from build123d import *

# Parameters (mm, degrees)
SKETCH1_R           = 30
SKETCH1_R_2         = 10
BOSS_EXTRUDE1_DEPTH = 6
CUT_EXTRUDE1_START  = -6
CUT_EXTRUDE1_DEPTH  = 6
CIRPATTERN1_COUNT   = 14


with BuildPart() as part:
    # Sketch1 → Boss-Extrude1 (new body)
    with BuildSketch(Plane.XY):
        Circle(SKETCH1_R)
        Circle(SKETCH1_R_2, mode=Mode.SUBTRACT)
    extrude(amount=BOSS_EXTRUDE1_DEPTH)

    # Sketch2 → Cut-Extrude1 (cut)
    with BuildSketch(Plane.XY.offset(6).offset(CUT_EXTRUDE1_START)):
        with BuildLine():
            Line((-4.028701623, 29.728262028), (-1.799877236, 25.12796678))
            ThreePointArc((-1.799877236, 25.12796678), (0, 24), (1.799877236, 25.12796678))
            Line((1.799877236, 25.12796678), (4.028701623, 29.728262028))
            ThreePointArc((4.028701623, 29.728262028), (0, 30), (-4.028701623, 29.728262028))
        make_face()
    cut_extrude1 = extrude(amount=CUT_EXTRUDE1_DEPTH, mode=Mode.SUBTRACT)

    # CirPattern1: Cut-Extrude1 ×14 about axis
    cirpattern1_axis = Axis((0, 0, 0), (0, 0, 1))
    for i in range(1, CIRPATTERN1_COUNT):
        add(cut_extrude1.rotate(cirpattern1_axis, i * 360 / CIRPATTERN1_COUNT), mode=Mode.SUBTRACT)


solid = part.part
Geometry check sheet. Reference: the model listing, model coordinates, mm. A direction names the side the tool comes from. Round coordinates to 2 decimals unless told otherwise and drop trailing zeros. Loops run counter-clockwise (first coordinate to the right, second up) from the corner with the lowest first, then second, coordinate; pieces in that order, holes last.
Item 1: Thickness scan on line 1 (Y direction, x = -27, z = 1.6); line 2 (Y direction, x = 0, z = 1.65); line 3 (Y direction, x = 24.5, z = 4.7). Record the ranges inside material, lowest first.
Item 2: Cross-section at B-B on y = 0. Record the boundary of the cut face in (x, z), then the cut area to 3 significant figures.
Item 3: Mould release check, pull along Y, two halves, no side actions. Record for faces 1 (the cylindrical face through (18.734, 23.431, 2.958)), 2 (the cylindrical face through (-6.71, -29.24, 2.96)), 3 (the flat face through (-27.35, -3.27, 2.96)): pulls with the +Y half, pulls with the -Y half, needs draft (parallel to the pull), parting line crosses it, or undercut.
Item 4: Access from +Z, -Z, +X, -X, +Y, -Y to the whole of each face (thin tool, end or side, straight path). Record for faces 4 (the flat face through (2.93, -27.46, 2.96)), 5 (the flat face through (-14.554, 23.47, 2.958)), 6 (the cylindrical face through (-18.675, 23.478, 2.958)), 7 (the flat face through (27.35, 3.27, 2.96)), 8 (the flat face through (-26.12, -8.967, 2.958)).
Item 5: Cross-section at A-A on x = 0. Record the boundary of the cut face in (y, z).
Item 6: Gauge pin test, flat ends, axial feed: pin 1 (1.5 mm diameter, centred on y = -12.5, z = 1.5, fed in from +X); pin 2 (3 mm diameter, centred on x = 20, z = 1, fed in from +Y); pin 3 (1 mm diameter, centred on x = -17.5, z = 1.5, fed in from +Y). Record the tip position at first contact, or that the pin passes through.
Answer sheet:
1. line 1: y = -13.08 to -9.67, -3.35 to 3.35, 9.67 to 13.08
1. line 2: y = -24 to -10, 10 to 24
1. line 3: y = -15.1 to -7.67, -3.97 to 3.97, 7.67 to 15.1
2. outline: (-30, 0) - (-10, 0) - (-10, 6) - (-30, 6) - close; (10, 0) - (30, 0) - (30, 6) - (10, 6) - close
2. area: 240 mm2
3. face 1: pulls with the +Y half
3. face 2: pulls with the -Y half
3. face 3: undercut
4. face 4: +Z, -Z, -Y
4. face 5: +Z, -Z, +Y
4. face 6: +Z, -Z, -X, +Y
4. face 7: +Z, -Z, +X
4. face 8: +Z, -Z, -X
5. outline: (-24, 0) - (-10, 0) - (-10, 6) - (-24, 6) - close; (10, 0) - (24, 0) - (24, 6) - (10, 6) - close
6. pin 1: stops at x = 27.6
6. pin 2: stops at y = 23.62
6. pin 3: stops at y = 24.72
